Input: part model. Units: mm. Frame: model coordinates. Round coordinates to 2 decimals unless told otherwise and drop trailing zeros. Loops run counter-clockwise (first coordinate to the right, second up) from the corner with the lowest first, then second, coordinate; pieces in that order, holes last.
1) Draft query along Y for faces 1 (the face through (0, 6, -10)), 2 (the face through (-55.06, 6.3, -31.37)), 3 (the face through (-38, 12.7, -10)). Return one class per face: pulls with the +Y half, pulls with the -Y half, needs draft (parallel to the pull), parting line crosses it, or undercut.
2) Section D-D, the plane z = -5. Return loops of the section in (x, y).
3) Section B-B, the plane x = -38.1. Return loops of the section in (y, z).
4) First-contact query: pin 1 (1.5 mm diameter, centred on y = 3, z = -21.5, fed in from +X); pin 2 (5 mm diameter, centred on y = 9.5, z = -21, fed in from +X); pin 3 (6 mm diameter, centred on x = -60, y = 7.5, fed in from -Z); pin 4 (1.5 mm diameter, centred on x = -54, y = 7.5, fed in from -Z). Flat tips, straight axial feed; report the tip coordinate or a pass-through.
5) Ray query, line 1 along Z through (x, y) = (-38.1, 4.25); line 2 along Y through (x, z) = (-19.05, -11); line 3 along X through (y, z) = (7, -20.5). Return the intervals inside material, ascending.
6) Section A-A, the plane z = -21.5. Return loops of the section in (x, y), and give its area (3 significant figures).
7) Section C-C, the plane y = 6.35. State how many separate pieces and enclosed holes the cut face has, and give its area (3 significant figures).
from build123d import *

# Parameters (mm, degrees)
BOSS_EXTRUDE1_DEPTH                               = 12.7
F_5_8_0_6250_DOWEL_HOLE2_D                        = 15.875
CSK_FOR_6_FLAT_HEAD_MACHINE_SCREW_100_D           = 3.6576
CSK_FOR_6_FLAT_HEAD_MACHINE_SCREW_100_CSINK_D     = 7.0866
CSK_FOR_6_FLAT_HEAD_MACHINE_SCREW_100_CSINK_ANGLE = 100


with BuildPart() as part:
    # Sketch2 → Boss-Extrude1 (new body)
    with BuildSketch(Plane(origin=(0, 0, 0), x_dir=(1, 0, 0), z_dir=(0, 1, 0))):
        with BuildLine():
            Line((0, 0), (-76.2, 0))
            Line((-76.2, 0), (-76.2, 19.05))
            ThreePointArc((-76.2, 19.05), (-38.1, 34.831536726), (0, 19.05))
            Line((0, 19.05), (0, 0))
        make_face()
    extrude(amount=BOSS_EXTRUDE1_DEPTH)

    # 5/8 (0.6250) Dowel Hole2 (through all)
    with Locations(Plane(origin=(0, 12.7, 0), x_dir=(1, 0, 0), z_dir=(0, 1, 0))):
        with Locations((-38.1, 19.05)):
            Hole(F_5_8_0_6250_DOWEL_HOLE2_D / 2)

    # CSK for #6 Flat Head Machine Screw (100)3 (through all)
    with Locations(Plane(origin=(0, 0, -32.5882), x_dir=(1, 0, 0), z_dir=(0, 0, -1))):
        with Locations((-19.05, -6.35), (-57.15, -6.35)):
            CounterSinkHole(CSK_FOR_6_FLAT_HEAD_MACHINE_SCREW_100_D / 2, CSK_FOR_6_FLAT_HEAD_MACHINE_SCREW_100_CSINK_D / 2, counter_sink_angle=CSK_FOR_6_FLAT_HEAD_MACHINE_SCREW_100_CSINK_ANGLE)


solid = part.part
Final values:
1. face 1: needs draft
1. face 2: undercut
1. face 3: pulls with the +Y half
2. outline: (-76.2, 0) - (0, 0) - (0, 12.7) - (-76.2, 12.7) - close; hole circle Ø3.66 at (-57.15, 6.35); hole circle Ø3.66 at (-19.05, 6.35)
3. outline: (0, -34.83) - (12.7, -34.83) - (12.7, -26.99) - (0, -26.99) - close; (0, -11.11) - (12.7, -11.11) - (12.7, 0) - (0, 0) - close
4. pin 1: stops at x = -1.78
4. pin 2: stops at x = 0
4. pin 3: stops at z = -31.35
4. pin 4: stops at z = -32.66
5. line 1: z = -34.83 to -26.99, -11.11 to 0
5. line 2: y = 0 to 4.52, 8.18 to 12.7
5. line 3: x = -74.69 to -58.86, -55.44 to -45.9, -30.3 to -20.76, -17.34 to -1.51
6. outline: (-73.58, 0) - (-45.65, 0) - (-45.65, 12.7) - (-73.58, 12.7) - close; (-30.55, 0) - (-2.62, 0) - (-2.62, 12.7) - (-30.55, 12.7) - close; hole circle Ø3.66 at (-57.15, 6.35); hole circle Ø3.66 at (-19.05, 6.35)
6. area: 688 mm2
7. separate pieces: 3
7. enclosed holes: 1
7. area: 1,850 mm2
